The figure shows three views and two pictorial views of one solid part (mm, origin at its lowest corner). Answer the questions. Give positions to 0.01 mm unless a question says otherwise; leave off trailing zeros. Order: outer loops, then holes, each group sorted by start corner. A loop starts at its lowest first (then second) coordinate and runs counter-clockwise, first axis right, second up. Notation, with made-up numbers: (62, 22) -> (81, 22) arc R23 cw to (81, 60) -> close; hole circle Ø10 at (-13.75, 14.25). An arc over 180 degrees is marked (long way). Use one line per item in the form item = value.
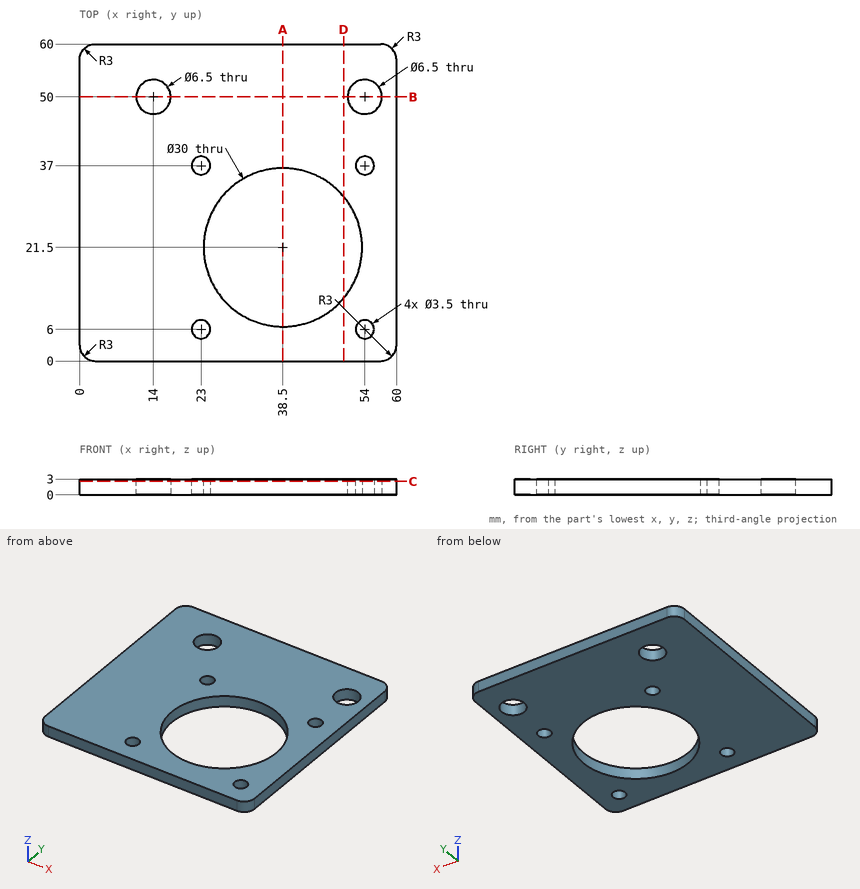
Item 1: The part is cut by section D-D on x = 50. Give the vertices of the cut face in (y, z), and give its area (3 significant figures).
Checks:
outline = (0, 0) -> (11.87, 0) -> (11.87, 3) -> (0, 3) -> close; (31.13, 0) -> (60, 0) -> (60, 3) -> (31.13, 3) -> close
area = 122 mm²
Item 2: The part is cut by section A-A on x = 38.5. Give the vertices of the cut face in (y, z).
Checks:
outline = (0, 0) -> (6.5, 0) -> (6.5, 3) -> (0, 3) -> close; (36.5, 0) -> (60, 0) -> (60, 3) -> (36.5, 3) -> close
Item 3: Straight lines are drawn through the part: L1, parallel to Y at x = 23, z = 1.2; L2, parallel to X at y = 51.5, z = 2.1; L3, parallel to Y at x = 14, z = 1.2. For each, find the intervals that lie inside material, in ascending order. Write a range as from..to.
Checks:
L1 = 0..4.25, 7.75..35.25, 38.75..60
L2 = 0..11.12, 16.88..51.12, 56.88..60
L3 = 0..46.75, 53.25..60
Item 4: The part is cut by section B-B on y = 50. Give the vertices of the cut face in (x, z), and give its area (3 significant figures).
Checks:
outline = (0, 0) -> (10.75, 0) -> (10.75, 3) -> (0, 3) -> close; (17.25, 0) -> (50.75, 0) -> (50.75, 3) -> (17.25, 3) -> close; (57.25, 0) -> (60, 0) -> (60, 3) -> (57.25, 3) -> close
area = 141 mm²
Item 5: The part is cut by section C-C on z = 2.55. Give the vertices of the cut face in (x, y).
Checks:
outline = (0, 3) arc R3 ccw to (3, 0) -> (57, 0) arc R3 ccw to (60, 3) -> (60, 57) arc R3 ccw to (57, 60) -> (3, 60) arc R3 ccw to (0, 57) -> close; hole circle Ø6.5 at (14, 50); hole circle Ø3.5 at (23, 6); hole circle Ø3.5 at (23, 37); hole circle Ø30 at (38.5, 21.5); hole circle Ø6.5 at (54, 50); hole circle Ø3.5 at (54, 6); hole circle Ø3.5 at (54, 37)
Item 6: Given pin 1 Ø6 at (x, y) = (14, 50) entering from -Z; pin 2 Ø1.5 at (x, z) = (53, 0.5) entering from -Y, each flat-ended and moving along its own axis, determine where each tip first touches the part or whether it passes through.
Checks:
pin_1 = through
pin_2 = 0
